Model file for the job. Use its own axes, mm. A direction names the side the tool comes from. Give positions to 0.01 mm unless a question says otherwise; leave off trailing zeros. Write each loop counter-clockwise with the first axis right and the second up, starting at its lowest first coordinate (ties: lowest second). Pieces come first, ordered by that corner, then holes. Notation, with made-up numbers: (22.25, 60) - (70.25, 60) arc R30 ccw to (70.25, 99) - close; hole circle Ø3 at (-6.5, -10). An arc over 180 degrees is marked (long way). Use CSV: the item, a comma, the result in double quotes.
Autodesk Inventor part; units mm, degrees
ref_plane "YZ Plane" through (0, 0, 0) normal (1, 0, 0) x (0, 1, 0)
ref_plane "XZ Plane" through (0, 0, 0) normal (0, 1, 0) x (-1, 0, 0)
ref_plane "XY Plane" through (0, 0, 0) normal (0, 0, 1) x (1, 0, 0)
sketch "Schizzo1" plane through (0, 0, 0) normal (0, 0, 1) x (1, 0, 0)
  line L0 (0, 0) -> (5, 0)
  line L1 (5, 0) -> (5, 40)
  line L2 (5, 40) -> (5.75, 40)
  line L3 (5.75, 40) -> (5.75, 84)
  line L4 (5.75, 84) -> (8.5, 84)
  line L5 (8.5, 84) -> (8.5, 96)
  line L6 (8.5, 96) -> (15, 96)
  line L7 (15, 96) -> (15, 99)
  line L8 (15, 99) -> (13.45, 99)
  line L9 (13.45, 99) -> (13.45, 102)
  line L10 (13.45, 102) -> (15, 102)
  line L11 (15, 102) -> (15, 106)
  line L12 (15, 106) -> (5, 106)
  line L13 (5, 106) -> (5, 104)
  line L14 (5, 104) -> (5.2, 104)
  line L15 (5.2, 104) -> (5.2, 102.9)
  line L16 (5.2, 102.9) -> (5, 102.9)
  line L17 (5, 102.9) -> (5, 96)
  line L18 (5, 96) -> (2.8047, 93.8047)
  line L19 (2.8047, 93.8047) -> (2.8047, 82)
  line L20 (2.8047, 82) -> (0, 80.3148)
  line L21 (0, 80.3148) -> (0, 0)
  dimension "d1" = 10
  dimension "d2" = 11.5
  dimension "d3" = 30
  dimension "d4" = 26.9
  dimension "d5" = 10.4
  dimension "d6" = 10
  dimension "d7" = 5.6094
  dimension "d8" = 17
  dimension "d9" = 40
  dimension "d10" = 84
  dimension "d11" = 96
  dimension "d12" = 10
  dimension "d13" = 4
  dimension "d14" = 3
  dimension "d15" = 2
  dimension "d16" = 1.1
  dimension "d17" = 45
  dimension "d18" = 59
  dimension "d19" = 24
revolve "Rivoluzione1" add sketch "Schizzo1" angle 360 about axis through (0, 80.3148, 0) along (0, -1, 0)
sketch "Schizzo2" plane through (0, 0, 0) normal (0, 0, 1) x (1, 0, 0)
  circle A0 centre (0, 91.5) radius 2.5
  line L0 (-15, 96) -> (15, 96)
  point P0 (0, 0)
  dimension "d21" = 5
  dimension "d22" = 4.5
extrude "Estrusione1" cut sketch "Schizzo2" along normal mid plane 30
sketch "Schizzo3" plane through (0, 0, 0) normal (0, -1, 0) x (1, 0, 0)
  line L0 (-4, 3) -> (-4, -3)
  line L1 (4, 3) -> (4, -3)
  circle A0 centre (0, 0) radius 5
  dimension "d25" = 1
extrude "Estrusione2" cut sketch "Schizzo3" against normal blind 14 contours L0 A0 | A0 L1
sketch "Schizzo4" plane through (4, 0, 3) normal (1, 0, 0) x (0, 0, -1)
  line L0 (6, 0) -> (0, 0)
  point P0 (3, 0)
  point P1 (3, 5)
  point P2 (3, 0)
  dimension "d30" = 5
hole "Foro1" at (4, 5, 0) direction (-1, 0, 0) diameter 5 end through all
properties part number "04-03-2023"
(1) Saw through at D-D, the plane y = 68. List the corners of the cut face in (x, z), then the cut area to 3 significant figures.
Checked values:
outline,"circle Ø11.5 at (0, 0)"
area,"104 mm^2"
(2) Saw through at C-C, the plane y = 91.5. List the corners of the cut face in (x, z), then the cut area to 3 significant figures.
Checked values:
outline,"(-2.5, -8.12) - (-2.5, -1.27) arc R2.8 cw to (-2.5, 1.27) - (-2.5, 8.12) arc R8.5 ccw to start; (2.5, -8.12) arc R8.5 ccw to (2.5, 8.12) - (2.5, 1.27) arc R2.8 cw to (2.5, -1.27) - close"
area,"142 mm^2"
(3) Flat gauge pins, fed straight in: P1, Ø3, axis at y = 18.5, z = -5.5, coming from the +X side; P2, Ø6.5, axis at y = 4, z = 0.5, coming from the -X side; P3, Ø6, axis at y = 68.5, z = 5, coming from the -X side. Where does each tip first touch, or does it go through?
Checked values:
P1,"stops at x = 3"
P2,"stops at x = -4"
P3,"stops at x = -5.39"
(4) Wall check: probe 1 along Y at (x, z) = (13.5, 0); probe 2 along Z at (x, y) = (0, 103.35); probe 3 along Y at (x, z) = (13, -0.25). Give the ranges that are in metal, low to high. Write a range as [from, to].
Checked values:
probe 1,"y = [96, 99], [102, 106]"
probe 2,"z = [-15, -5.2], [5.2, 15]"
probe 3,"y = [96, 106]"
(5) Pull direction Y, two halves, no side cores. Call faces 5 (the face through (1.358, 93.942, 2.61)), 6 (the face through (0, 0, 0)), 7 (the face through (-0.677, 103.442, 5.156)): released by +Y, released by -Y, zero draft, split by the parting line, or undercut.
Checked values:
face 5,"released by +Y"
face 6,"released by -Y"
face 7,"undercut"
(6) 3-axis set-ups, long thin cutter, end or side, ignore diameter. For faces 1 (the face through (-2, 40, 5)), 2 (the face through (4, 8, 0)), 3 (the face through (-3.4, 102, 13.4)), 4 (the face through (2.675, 86.508, 0.842)): which of +Z, -Z, +X, -X, +Y, -Y reach the whole face in a straight line?
Checked values:
face 1,"-Y"
face 2,"+Z, -Z, +X, -Y"
face 3,"none"
face 4,"+Y"
(7) Saw through at B-B, the plane y = 37.5. List the corners of the cut face in (x, z), then the cut area to 3 significant figures.
Checked values:
outline,"circle Ø10 at (0, 0)"
area,"78.5 mm^2"
(8) Saw through at A-A, the plane y = 5. List the corners of the cut face in (x, z).
Checked values:
outline,"(-4, -3) arc R5 ccw to (4, -3) - (4, -2.5) - (-4, -2.5) - close; (-4, 2.5) - (4, 2.5) - (4, 3) arc R5 ccw to (-4, 3) - close"
